Source: three-view drawing plus pictorial views. Frame: mm from the lowest corner of the part. A direction names the side the tool comes from. Round coordinates to 2 decimals unless told otherwise and drop trailing zeros. Loops run counter-clockwise (first coordinate to the right, second up) from the corner with the lowest first, then second, coordinate; pieces in that order, holes last. Notation, with made-up numbers: (14, -19.5) -> (30, -19.5) arc R21 cw to (30, -4.5) -> close; hole circle Ø11 at (-34, 3). An arc over 180 degrees is marked (long way). Answer as a JSON object with one key per item and string values. Group by question number.
Item 1: Section query B-B on x = 40. Return loops of the section in (y, z).
Item 2: Set-up query: the marked faces 4, 5 and 6. Return all of +Z, -Z, +X, -X, +Y, -Y with unobstructed straight access to the full face (end or side cutting, diameter ignored); none if empty.
Item 3: Section query D-D on y = 67.5. Return loops of the section in (x, z).
Item 4: Section query C-C on z = 8. Return loops of the section in (x, y), and give its area (3 significant figures).
Item 5: Material intervals for line 1 (Y direction, x = 40, z = 3); line 2 (Y direction, x = 49, z = 36.5); line 3 (Z direction, x = 70.5, y = 15), sorted ascending. Write a range as [from, to].
Item 6: Draft query along X for the marked faces 1, 2 and 3. Return one class per face: released by +X, released by -X, zero draft, split by the parting line, or undercut.
Item 7: Section query A-A on y = 40. Return loops of the section in (x, z), and give its area (3 significant figures).
Item 8: Pin query (flat end, axial travel): pin 1 (22 mm diameter, centred on x = 42.5, z = 37, fed in from +Y); pin 2 (2.5 mm diameter, centred on y = 76.5, z = 33.5, fed in from +X); pin 3 (10 mm diameter, centred on x = 44.5, z = 38, fed in from -Y). Return the tip coordinate at first contact, or that it passes through.
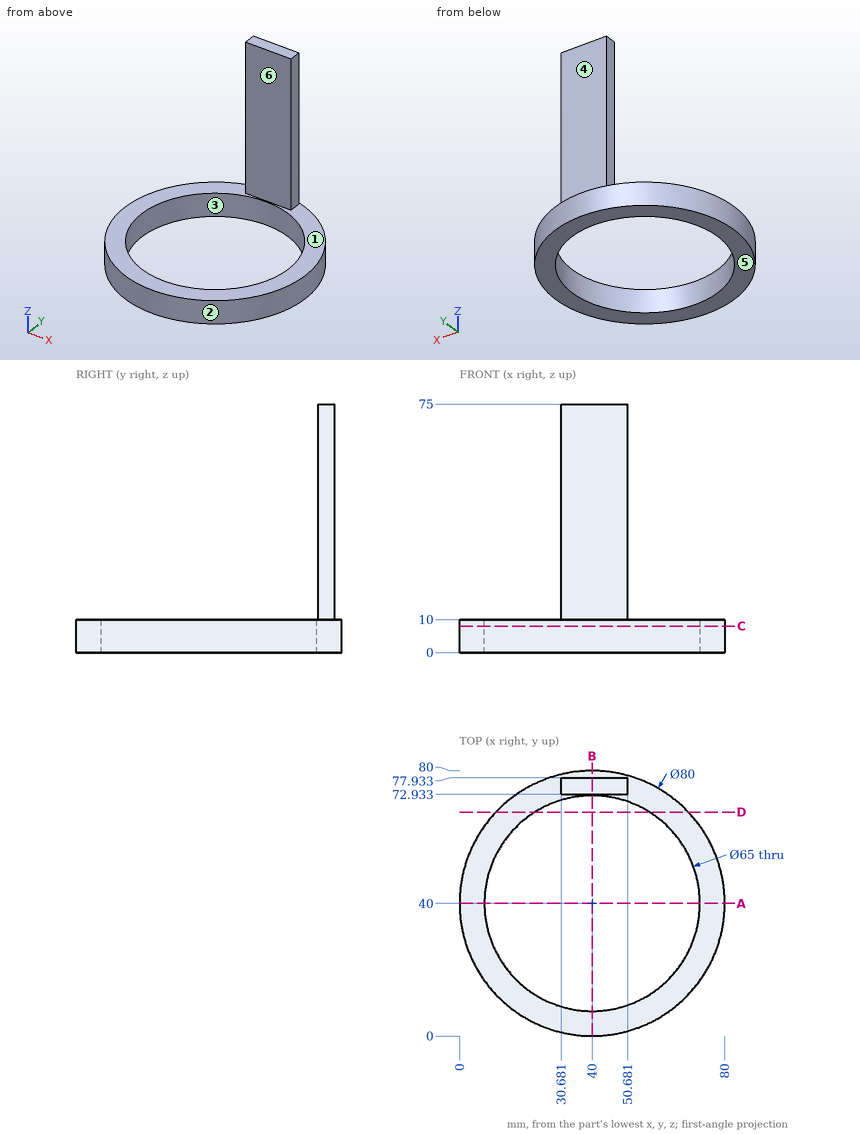
Solved:
{
 "1": {"outline": "(0, 0) -> (7.5, 0) -> (7.5, 10) -> (0, 10) -> close; (72.5, 0) -> (80, 0) -> (80, 10) -> (77.93, 10) -> (77.93, 75) -> (72.93, 75) -> (72.93, 10) -> (72.5, 10) -> close"},
 "2": {"face 4": "+Z, +X, -X, +Y", "face 5": "-Z, +X, -X, +Y, -Y", "face 6": "+Z, +X, -X, -Y"},
 "3": {"outline": "(10.95, 0) -> (22.68, 0) -> (22.68, 10) -> (10.95, 10) -> close; (57.32, 0) -> (69.05, 0) -> (69.05, 10) -> (57.32, 10) -> close"},
 "4": {"outline": "circle Ø80 at (40, 40); hole circle Ø65 at (40, 40)", "area": "1,710 mm²"},
 "5": {"line 1": "[0, 7.5], [72.5, 80]", "line 2": "[72.93, 77.93]", "line 3": "[0, 10]"},
 "6": {"face 1": "zero draft", "face 2": "split by the parting line", "face 3": "undercut"},
 "7": {"outline": "(0, 0) -> (7.5, 0) -> (7.5, 10) -> (0, 10) -> close; (72.5, 0) -> (80, 0) -> (80, 10) -> (72.5, 10) -> close", "area": "150 mm²"},
 "8": {"pin 1": "y = 77.93", "pin 2": "x = 50.68", "pin 3": "y = 72.93"}
}
